```python
from build123d import *

# Parameters (mm, degrees)
F1_DEPTH = 19.05
F2_R     = 101.6
F3_R     = 1270
F4_R     = 12.827
F5_DEPTH = 19.051


# Not quite as in the source:
# - a feature names something its author has since deleted; it is built from what else it names


with BuildPart() as f1:
    # F0 (on Top) → F1 (new body)
    with BuildSketch(Plane.XY):
        Polygon((-304.8, 0), (0, 0), (304.8, 0), (406.4, 1270), (373.888, 1676.4), (0, 1676.4), (-373.888, 1676.4), (-406.4, 1270), align=None)
        Polygon((-326.989699267, 1625.6), (0, 1625.6), (326.989699267, 1625.6), (355.437699267, 1270), (257.901699267, 50.8), (0, 50.8), (-257.901699267, 50.8), (-355.437699267, 1270), align=None, mode=Mode.SUBTRACT)
    extrude(amount=F1_DEPTH)

    # F2
    f2_edges = [f1.edges().sort_by_distance(p)[0] for p in [
        (-304.8, 0, 9.525),
        (304.8, 0, 9.525),
        (373.888, 1676.4, 9.525),
        (-373.888, 1676.4, 9.525),
        (-326.989699, 1625.6, 9.525),
        (326.989699, 1625.6, 9.525),
        (-257.901699, 50.8, 9.525),
        (257.901699, 50.8, 9.525),
    ]]
    fillet(f2_edges, radius=F2_R)

    # F3
    f3_edges = [f1.edges().sort_by_distance(p)[0] for p in [
        (-406.4, 1270, 9.525),
        (406.4, 1270, 9.525),
    ]]
    fillet(f3_edges, radius=F3_R)

    # F4 (on face) → F5 (cut, through all)
    with BuildSketch(Plane.XY.offset(19.05)):
        with Locations((256.4722616265, 52.3483595568)):
            Circle(F4_R)
        with Locations((-256.4722616265, 52.3483595568)):
            Circle(F4_R)
        with Locations((-325.5602616265, 1624.0516404432)):
            Circle(F4_R)
        with Locations((325.5602616265, 1624.0516404432)):
            Circle(F4_R)
    extrude(amount=-F5_DEPTH, mode=Mode.SUBTRACT)


solid = f1.part
```
Input: part model. Units: mm. Frame: model coordinates. A direction names the side the tool comes from. Coordinates: 2 decimals unless noted, no trailing zeros. Loops run counter-clockwise (first coordinate to the right, second up) from the corner with the lowest first, then second, coordinate; pieces in that order, holes last. Notation, with made-up numbers: M -31.75,-23 L 15.25,-23 A14 cw 15.25,-3 Z; hole C 65.25,10 d10. An arc over 180 degrees is marked long. Use a Markdown table: item, result. Add a question column.
1) Pin query (flat end, axial travel): P1, Ø10, axis at x = 316, y = 859, coming from the -Z side; P2, Ø4, axis at y = 519.5, z = 3.5, coming from the -X side; P3, Ø4, axis at y = 1119, z = 9, coming from the -X side; P4, Ø6, axis at y = 722, z = 11, coming from the -X side. Return the tip coordinate at first contact, or that it passes through.
2) Section A-A, the plane x = 17. Return the cut outline in (y, z).
3) Section B-B, the plane y = 583. Return the cut outline in (x, z), plus the area to 3 significant figures.
4) Line query: L1, parallel to Y at x = -86, z = 10.5; L2, parallel to X at y = 1198.5, z = 1; L3, parallel to Y at x = 187.5, z = 2.5. Output: solid intervals per line, ascending. Write a range as from..to.
5) Draft query along X for faces 1 (the flat face through (-330, 904, 0)), 2 (the cylindrical face through (-348.227, 1650.167, 9.658)), 3 (the flat face through (354.687, 623.584, 9.392)), 4 (the flat face through (-309.78, 699.27, 9.39)). Return one class per face: +X half, -X half, draft (parallel to the pull), parting line (faces both ways), or undercut.
6) Set-up query: faces 5 (the flat face through (311.04, 715.03, 9.39)), 6 (the cylindrical face through (349.785, 1648.728, 9.658)). Return all of +Z, -Z, +X, -X, +Y, -Y with unobstructed straight access to the full face (end or side cutting, diameter ignored); none if empty.
7) Section C-C, the plane z = 8.25. Return the cut outline in (x, y), plus the area to 3 significant figures.
Answer below:
| question | item | result |
|---|---|---|
| 1 | P1 | through |
| 1 | P2 | x = -346.52 |
| 1 | P3 | x = -394.48 |
| 1 | P4 | x = -362.8 |
| 2 | outline | M 0,0 L 50.8,0 L 50.8,19.05 L 0,19.05 Z; M 1625.6,0 L 1676.4,0 L 1676.4,19.05 L 1625.6,19.05 Z |
| 3 | outline | M -351.44,0 L -300.48,0 L -300.48,19.05 L -351.44,19.05 Z; M 300.48,0 L 351.44,0 L 351.44,19.05 L 300.48,19.05 Z |
| 3 | area | 1,940 mm2 |
| 4 | L1 | 0..50.8, 1625.6..1676.4 |
| 4 | L2 | -400.33..-349.72, 349.72..400.33 |
| 4 | L3 | 0..53.53, 1625.6..1676.4 |
| 5 | face 1 | draft |
| 5 | face 2 | -X half |
| 5 | face 3 | +X half |
| 5 | face 4 | undercut |
| 6 | face 5 | +Z, -Z |
| 6 | face 6 | +Z, -Z, +X, +Y |
| 7 | outline | M -398.3,1168.72 L -312.28,93.5 A101.6 ccw -211,0 L 211,0 A101.6 ccw 312.28,93.5 L 398.3,1168.72 A1270 ccw 398.3,1371.28 L 381.37,1582.9 A101.6 ccw 280.09,1676.4 L -280.09,1676.4 A101.6 ccw -381.37,1582.9 L -398.3,1371.28 A1270 ccw Z; hole M -355.44,1270 L -265.38,144.3 A101.6 ccw -164.11,50.8 L 164.11,50.8 A101.6 ccw 265.38,144.3 L 355.44,1270 L 334.47,1532.1 A101.6 ccw 233.19,1625.6 L -233.19,1625.6 A101.6 ccw -334.47,1532.1 Z; hole C -325.56,1624.05 d25.65; hole C -256.47,52.35 d25.65; hole C 256.47,52.35 d25.65; hole C 325.56,1624.05 d25.65 |
| 7 | area | 227,000 mm2 |
